Here's how the part is built. I have some questions about the finished solid (model axes, mm). A direction names the side the tool comes from. Round coordinates to 2 decimals unless told otherwise and drop trailing zeros. Loops run counter-clockwise (first coordinate to the right, second up) from the corner with the lowest first, then second, coordinate; pieces in that order, holes last. Notation, with made-up numbers: M 9.25,-24 L 51.25,-24 A17 cw 51.25,-6 Z; hole C 24,63 d7. An arc over 180 degrees is marked long. Answer as CSV lines item,"result".
```python
from build123d import *

# Parameters (mm, degrees)
SKETCH2_W            = 40.2336
SKETCH2_H            = 25.019
SKETCH2_R            = 1.05
BOSS_EXTRUDE1_DEPTH  = 1.5
BOSS_EXTRUDE2_DEPTH  = 6.35
SKETCH4_R            = 8
BOSS_EXTRUDE3_DEPTH  = 9.2
SKETCH5_R            = 5.95
BOSS_EXTRUDE4_DEPTH  = 2.36
SKETCH6_R            = 8.5217
LENS_DEPTH           = 4
SKETCH7_W            = 4.22
SKETCH7_H            = 7.75
BOSS_EXTRUDE6_DEPTH  = 8.3
SKETCH8_W            = 9
SKETCH8_H            = 2.93
BOSS_EXTRUDE7_DEPTH  = 4.35
SKETCH9_W            = 3.1
SKETCH9_H            = 5
BOSS_EXTRUDE8_DEPTH  = 1.3
SKETCH10_W           = 25.5
SKETCH10_H           = 8
BOSS_EXTRUDE9_DEPTH  = 1.4
SKETCH11_W           = 1.3
SKETCH11_H           = 2
BOSS_EXTRUDE10_DEPTH = 1.6
SKETCH12_W           = 3
SKETCH12_H           = 3
BOSS_EXTRUDE11_DEPTH = 1.4
SKETCH13_W           = 3.175
SKETCH13_H           = 2.6162
SKETCH13_W_2         = 8.509
SKETCH13_H_2         = 4.826
BOSS_EXTRUDE12_DEPTH = 2.7432
DOME1_FACE_RADIUS    = 8.5217
DOME1_HEIGHT         = 2.54


with BuildPart() as part:
    # Sketch2 → Boss-Extrude1 (new body)
    with BuildSketch(Plane.XY):
        Rectangle(SKETCH2_W, SKETCH2_H)
        with Locations((-18.4568, 10.8495)):
            Circle(SKETCH2_R, mode=Mode.SUBTRACT)
        with Locations(Location((-18.4568, -10.8495, 0), (0, 0, 180))):
            Circle(SKETCH2_R, mode=Mode.SUBTRACT)
        with Locations((18.4568, -10.8495)):
            Circle(SKETCH2_R, mode=Mode.SUBTRACT)
        with Locations(Location((18.4568, 10.8495, 0), (0, 0, 180))):
            Circle(SKETCH2_R, mode=Mode.SUBTRACT)
    extrude(amount=BOSS_EXTRUDE1_DEPTH)

    # Sketch3 → Boss-Extrude2 (add)
    with BuildSketch(Plane.XY.offset(1.5)):
        with BuildLine():
            Line((-8.4, -2.05), (-8.4, -8.4))
            Line((-8.4, -8.4), (8.4, -8.4))
            Line((8.4, -8.4), (8.4, -2.05))
            Line((8.4, -2.05), (10.7, -2.05))
            ThreePointArc((10.7, -2.05), (12.75, 0), (10.7, 2.05))
            Line((10.7, 2.05), (8.4, 2.05))
            Line((8.4, 2.05), (8.4, 8.4))
            Line((8.4, 8.4), (-8.4, 8.4))
            Line((-8.4, 8.4), (-8.4, 2.05))
            Line((-8.4, 2.05), (-10.7, 2.05))
            ThreePointArc((-10.7, 2.05), (-12.75, 0), (-10.7, -2.05))
            Line((-10.7, -2.05), (-8.4, -2.05))
        make_face()
    extrude(amount=BOSS_EXTRUDE2_DEPTH)

    # Sketch4 → Boss-Extrude3 (add)
    with BuildSketch(Plane.XY.offset(7.85)):
        Circle(SKETCH4_R)
    extrude(amount=BOSS_EXTRUDE3_DEPTH)

    # Sketch5 → Boss-Extrude4 (add)
    with BuildSketch(Plane.XY.offset(17.05)):
        Circle(SKETCH5_R)
    extrude(amount=BOSS_EXTRUDE4_DEPTH)

    # Sketch6 → Lens (add)
    with BuildSketch(Plane.XY.offset(19.41)):
        Circle(SKETCH6_R)
    extrude(amount=LENS_DEPTH)

    # Sketch7 → Boss-Extrude6 (add)
    with BuildSketch(Plane(origin=(0, 0, 0), x_dir=(-1, 0, 0), z_dir=(0, 0, -1))):
        with Locations((-17.5068, 0)):
            Rectangle(SKETCH7_W, SKETCH7_H)
    extrude(amount=BOSS_EXTRUDE6_DEPTH)

    # Sketch8 → Boss-Extrude7 (add)
    with BuildSketch(Plane(origin=(0, 0, 0), x_dir=(-1, 0, 0), z_dir=(0, 0, -1))):
        with Locations((11.1768, -9.4045)):
            Rectangle(SKETCH8_W, SKETCH8_H)
    extrude(amount=BOSS_EXTRUDE7_DEPTH)

    # Sketch9 → Boss-Extrude8 (add)
    with BuildSketch(Plane.XY.offset(1.5)):
        with Locations((13.0668, 8.5095)):
            Rectangle(SKETCH9_W, SKETCH9_H)
    extrude(amount=BOSS_EXTRUDE8_DEPTH)

    # Sketch10 → Boss-Extrude9 (add)
    with BuildSketch(Plane(origin=(0, 0, 0), x_dir=(-1, 0, 0), z_dir=(0, 0, -1))):
        with Locations((-0.3668, 8.2095)):
            Rectangle(SKETCH10_W, SKETCH10_H)
    extrude(amount=BOSS_EXTRUDE9_DEPTH)

    # Sketch11 → Boss-Extrude10 (add)
    with BuildSketch(Plane.XY.offset(1.5)):
        with Locations((14.7668, -9.5095)):
            Rectangle(SKETCH11_W, SKETCH11_H)
        with Locations((-17.777092667, 6.391636208)):
            Rectangle(SKETCH11_W, SKETCH11_H)
    extrude(amount=BOSS_EXTRUDE10_DEPTH)

    # Sketch12 → Boss-Extrude11 (add)
    with BuildSketch(Plane(origin=(0, 0, 0), x_dir=(-1, 0, 0), z_dir=(0, 0, -1))):
        with Locations((17.6168, 6.6095)):
            Rectangle(SKETCH12_W, SKETCH12_H)
    extrude(amount=BOSS_EXTRUDE11_DEPTH)

    # Sketch13 → Boss-Extrude12 (add)
    with BuildSketch(Plane(origin=(0, 0, 0), x_dir=(-1, 0, 0), z_dir=(0, 0, -1))):
        with Locations((-12.5603, -10.6934)):
            Rectangle(SKETCH13_W, SKETCH13_H)
        with Locations((-2.9083, -9.5885)):
            Rectangle(SKETCH13_W_2, SKETCH13_H_2)
    extrude(amount=BOSS_EXTRUDE12_DEPTH)

    # Dome1: a dome of height H over a round flat face of radius A is a cap of a sphere of radius (A * A + H * H) / (2 * H)
    dome1_r = (DOME1_FACE_RADIUS * DOME1_FACE_RADIUS + DOME1_HEIGHT * DOME1_HEIGHT) / (2 * DOME1_HEIGHT)
    dome1_base = Plane((0, 0, 23.41), z_dir=(0, 0, 1))
    with Locations(dome1_base.offset(DOME1_HEIGHT - dome1_r)):
        dome1_ball = Sphere(dome1_r, mode=Mode.PRIVATE)
    add(split(dome1_ball, bisect_by=dome1_base, keep=Keep.TOP, mode=Mode.PRIVATE))


solid = part.part
```
1. Which directions (+Z, -Z, +X, -X, +Y, -Y) give clear straight access to the entire face, cutting with the end or side of a thin tool? Please do faces 4 (the flat face through (-1.346, -10, -1)), 5 (the flat face through (3, -7.176, -1)), 6 (the flat face through (13.117, 8, -1)).
Evaluation:
face 4,"-Z, -Y"
face 5,"-Z, +X, -X"
face 6,"-Z, +X, +Y"
2. If I drill on line 1 (Z direction, x = -11.5, y = 3); line 2 (X direction, y = -7.25, z = 6), over which ranges is the centre line in solid material (lowest first)? Write a range as [from, to].
Evaluation:
line 1,"z = [0, 1.5]"
line 2,"x = [-8.4, 8.4]"
3. We'd pull the mould along Y, two halves only. Please class faces 1 (the flat face through (1, 12.21, -1)), 2 (the cylindrical face through (-17.892, 11.735, 0.74)), 3 (the flat face through (-6, -2, 19.41)): pulls with the +Y half, pulls with the -Y half, needs draft (parallel to the pull), parting line crosses it, or undercut.
Evaluation:
face 1,"pulls with the +Y half"
face 2,"undercut"
face 3,"needs draft"
4. I want a section at B-B, the plane y = 0. Please give me the cut outline in (x, z).
Evaluation:
outline,"M -20.12,0 L 15.4,0 L 15.4,-8.3 L 19.62,-8.3 L 19.62,0 L 20.12,0 L 20.12,1.5 L 12.75,1.5 L 12.75,7.85 L 8,7.85 L 8,17.05 L 5.95,17.05 L 5.95,19.41 L 8.52,19.41 L 8.52,23.41 A15.57 ccw -8.52,23.41 L -8.52,19.41 L -5.95,19.41 L -5.95,17.05 L -8,17.05 L -8,7.85 L -12.75,7.85 L -12.75,1.5 L -20.12,1.5 Z"
5. I want a section at C-C, the plane z = 16.5. Please give me the cut outline in (x, y), and give its area (3 significant figures).
Evaluation:
outline,"C 0,0 d16"
area,"201 mm²"
6. I want a section at D-D, the plane x = 0. Please give me the cut outline in (y, z), and give its area (3 significant figures).
Evaluation:
outline,"M -12.51,0 L -12,0 L -12,-2.74 L -7.18,-2.74 L -7.18,0 L 4.21,0 L 4.21,-1.4 L 12.21,-1.4 L 12.21,0 L 12.51,0 L 12.51,1.5 L 8.4,1.5 L 8.4,7.85 L 8,7.85 L 8,17.05 L 5.95,17.05 L 5.95,19.41 L 8.52,19.41 L 8.52,23.41 A15.57 ccw -8.52,23.41 L -8.52,19.41 L -5.95,19.41 L -5.95,17.05 L -8,17.05 L -8,7.85 L -8.4,7.85 L -8.4,1.5 L -12.51,1.5 Z"
area,"441 mm²"
7. I want a section at A-A, the plane x = -13.5. Please give me the cut outline in (y, z), and give its area (3 significant figures).
Evaluation:
outline,"M -12.51,0 L -10.87,0 L -10.87,-4.35 L -7.94,-4.35 L -7.94,0 L 12.51,0 L 12.51,1.5 L -12.51,1.5 Z"
area,"50.3 mm²"
8. For P1, Ø12, axis at y = 3, z = 9, coming from the +X side; P2, Ø3, axis at x = -4.5, z = -2.5, coming from the +Y side; P3, Ø1.5, axis at x = -3, y = -7.5, coming from the -Z side, each with a flat end and sliding along its axis, tell me the tip position at first contact or that it passes through.
Evaluation:
P1,"stops at x = 12.75"
P2,"stops at y = 12.21"
P3,"stops at z = 0"
